Model file for the job. Use its own axes, mm. A direction names the side the tool comes from. Coordinates: 2 decimals unless noted, no trailing zeros. Order: outer loops, then holes, each group sorted by start corner. A loop starts at its lowest first (then second) coordinate and runs counter-clockwise, first axis right, second up. Notation, with made-up numbers: (59, -6.5) -> (87, -6.5) arc R32 cw to (87, 19.5) -> close; hole circle Ø1 at (19, 79). An arc over 180 degrees is marked (long way). Use CSV: the item, a comma, the result in double quotes. Start each with the question number.
(1) Pull direction X, two halves, no side cores. Call faces 4 (the flat face through (-18.893, 9.86, 30.319)), 5 (the flat face through (7.232, 10, 66)), 6 (the cylindrical face through (0, 10, -20)): pulls with the +X half, pulls with the -X half, needs draft (parallel to the pull), parting line crosses it, or undercut.
(2) Probe L1, parallel to Z at x = -1.5, y = 55; L2, parallel to Z at x = -4.5, y = 22; L3, parallel to Y at x = 11, z = 40. List the from-to ranges inside material, lowest first.
(3) Cut at B-B on z = 48. Write the cut outline in (x, y).
(4) Cut at C-C on x = -6. Write the cut outline in (y, z), plus the area to 3 significant figures.
(5) Cut at D-D on y = 47.5. Write the cut outline in (x, z), plus the area to 3 significant figures.
(6) Tool access for faces 1 (the flat face through (-2.768, 10, 66)), 2 (the flat face through (-18.045, 45, 53)), 3 (the flat face through (-13, 10, 60.739)): list every direction of +Z, -Z, +X, -X, +Y, -Y with a clear straight run to the whole face (end or side of a thin tool).
(7) Cut at A-A on y = 19. Write the cut outline in (x, z), plus the area to 3 significant figures.
(8) Pin check, flat tips, straight feed: pin 1 Ø3 at (x, y) = (-15, 7.5) entering from +Z; pin 2 Ø3 at (y, z) = (10, 66.5) entering from -X; pin 3 Ø10 at (y, z) = (10.5, 60) entering from -X. Stop position of each tip, or through.
```python
from build123d import *

# Parameters (mm, degrees)
BOSS_EXTRUDE1_DEPTH = 20
SKETCH2_W           = 40
SKETCH2_H           = 5
BOSS_EXTRUDE2_DEPTH = 50
SKETCH3_R           = 10
BOSS_EXTRUDE3_DEPTH = 10


with BuildPart() as part:
    # Sketch1 → Boss-Extrude1 (new body)
    with BuildSketch(Plane(origin=(0, 0, 0), x_dir=(1, 0, 0), z_dir=(0, 1, 0))):
        with BuildLine():
            Line((22.186265925, -59.437832279), (19.9931848, 0.522074285))
            ThreePointArc((19.9931848, 0.522074285), (-0.630541833, 19.990057954), (-19.986342651, -0.738990821))
            Line((-19.986342651, -0.738990821), (-17.767855256, -60.738990821))
            Line((-17.767855256, -60.738990821), (-7.767855256, -60.738990821))
            Line((-7.767855256, -60.738990821), (-7.767855256, -70.738990821))
            Line((-7.767855256, -70.738990821), (-2.767855256, -70.738990821))
            Line((-2.767855256, -70.738990821), (-2.767855256, -60.738990821))
            Line((-2.767855256, -60.738990821), (7.232144744, -60.738990821))
            Line((7.232144744, -60.738990821), (7.232144744, -70.738990821))
            Line((7.232144744, -70.738990821), (12.232144744, -70.738990821))
            Line((12.232144744, -70.738990821), (12.232144744, -60.738990821))
            Line((12.232144744, -60.738990821), (22.232144744, -60.738990821))
            ThreePointArc((22.232144744, -60.738990821), (22.220671476, -60.088007254), (22.186265925, -59.437832279))
        make_face()
    extrude(amount=BOSS_EXTRUDE1_DEPTH)

    # Sketch2 → Boss-Extrude2 (add)
    with BuildSketch(Plane(origin=(0, 20, 0), x_dir=(1, 0, 0), z_dir=(0, 1, 0))):
        with Locations((1.954821984, -53.238670729)):
            Rectangle(SKETCH2_W, SKETCH2_H)
    extrude(amount=BOSS_EXTRUDE2_DEPTH)

    # Sketch3 → Boss-Extrude3 (add)
    with BuildSketch(Plane(origin=(0, -50, 50.738670729), x_dir=(-1, 0, 0), z_dir=(0, 0, -1))):
        with Locations(Location((-1.954821984, 102.596055016, 0), (0, 0, 180))):
            Circle(SKETCH3_R)
    extrude(amount=BOSS_EXTRUDE3_DEPTH)


solid = part.part
```
Outcome:
1,face 4,"pulls with the -X half"
1,face 5,"undercut"
1,face 6,"parting line crosses it"
2,L1,"40.74 to 55.74"
2,L2,"50.74 to 55.74"
2,L3,"0 to 20"
3,outline,"(-18.24, 0) -> (21.77, 0) -> (21.77, 20) -> (-18.24, 20) -> close; circle Ø20 at (1.95, 52.6)"
4,outline,"(0, -19.08) -> (20, -19.08) -> (20, 50.74) -> (46.54, 50.74) -> (46.54, 40.74) -> (58.66, 40.74) -> (58.66, 50.74) -> (70, 50.74) -> (70, 55.74) -> (20, 55.74) -> (20, 70.74) -> (0, 70.74) -> close"
4,area,"2,170 mm2"
5,outline,"(-18.05, 50.74) -> (-6.65, 50.74) -> (-6.65, 40.74) -> (10.56, 40.74) -> (10.56, 50.74) -> (21.95, 50.74) -> (21.95, 55.74) -> (-18.05, 55.74) -> close"
5,area,"372 mm2"
6,face 1,"+Z, +Y, -Y"
6,face 2,"+Z, -Z, -X, +Y"
6,face 3,"+Z, -X, +Y, -Y"
7,outline,"(-19.99, 0.74) arc R20 ccw (long way) to (19.99, -0.52) -> (22.19, 59.44) arc R18.47 ccw to (22.23, 60.74) -> (12.23, 60.74) -> (12.23, 70.74) -> (7.23, 70.74) -> (7.23, 60.74) -> (-2.77, 60.74) -> (-2.77, 70.74) -> (-7.77, 70.74) -> (-7.77, 60.74) -> (-17.77, 60.74) -> close"
7,area,"3,160 mm2"
8,pin 1,"z = 60.74"
8,pin 2,"x = -7.77"
8,pin 3,"x = -17.98"
